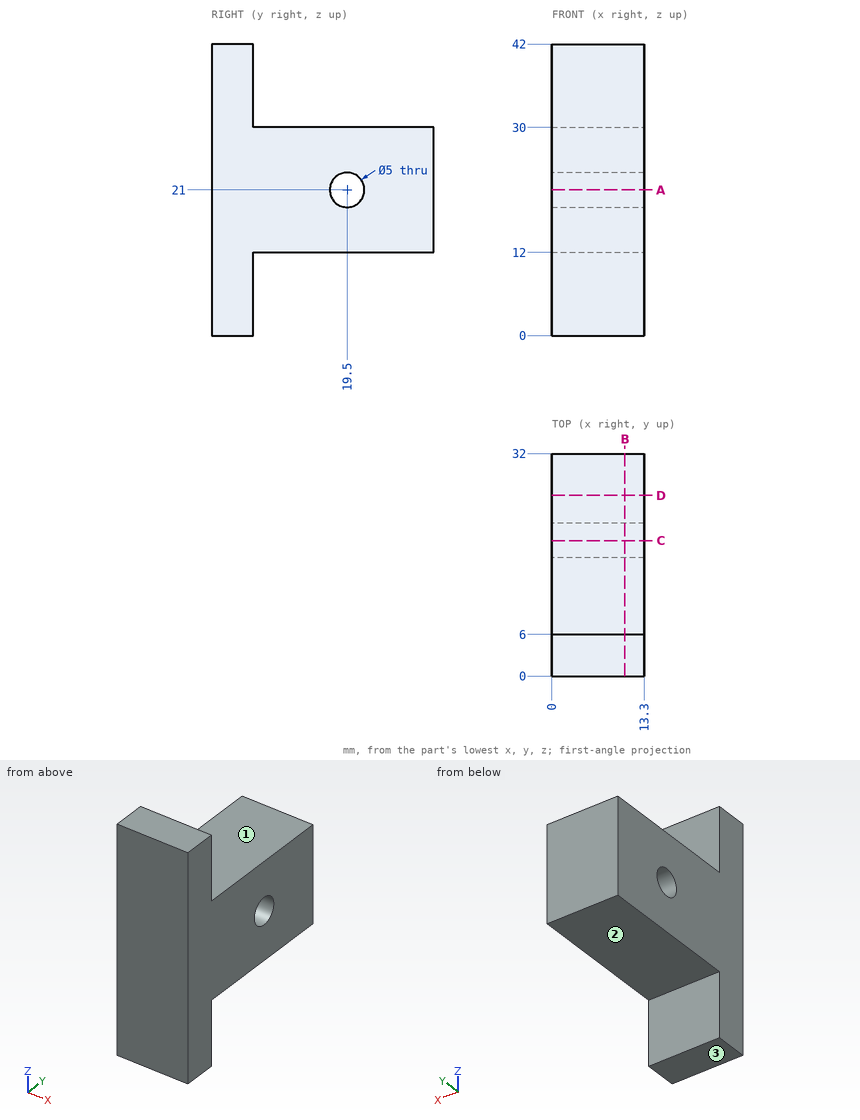
Part print with two shaded views. Sizes in mm from the minimum x, y, z corner. A direction names the side the tool comes from. Coordinates: 2 decimals unless noted, no trailing zeros. Write each loop counter-clockwise with the first axis right and the second up, starting at its lowest first coordinate (ties: lowest second). Pieces come first, ordered by that corner, then holes.
1. Band-saw the part on B-B, the plane x = 10.5. Give the cut face in (y, z).
Answer block:
outline: (0, 0) - (6, 0) - (6, 12) - (32, 12) - (32, 30) - (6, 30) - (6, 42) - (0, 42) - close; hole circle Ø5 at (19.5, 21)
2. Band-saw the part on A-A, the plane z = 21. Give the cut face in (x, y).
Answer block:
outline: (0, 0) - (13.3, 0) - (13.3, 17) - (0, 17) - close; (0, 22) - (13.3, 22) - (13.3, 32) - (0, 32) - close
3. Drop flat-ended pins along their axis: pin 1 (4 mm diameter, centred on y = 24.5, z = 33, fed in from -X); pin 2 (6 mm diameter, centred on x = 11.5, y = 10.5, fed in from +Z); pin 3 (1 mm diameter, centred on x = 2, y = 10, fed in from -Z); pin 4 (3.5 mm diameter, centred on x = 9.5, z = 4, fed in from +Y). Give the stop position or say it passes through.
Answer block:
pin 1: passes through
pin 2: stops at z = 30
pin 3: stops at z = 12
pin 4: stops at y = 6
4. 3-axis set-ups, long thin cutter, end or side, ignore diameter. For the marked faces 1, 2 and 3: which of +Z, -Z, +X, -X, +Y, -Y reach the whole face in a straight line?
Answer block:
face 1: +Z, +X, -X, +Y
face 2: -Z, +X, -X, +Y
face 3: -Z, +X, -X, +Y, -Y
5. Band-saw the part on C-C, the plane y = 19.5. Give the cut face in (x, z), and give its area (3 significant figures).
Answer block:
outline: (0, 12) - (13.3, 12) - (13.3, 18.5) - (0, 18.5) - close; (0, 23.5) - (13.3, 23.5) - (13.3, 30) - (0, 30) - close
area: 173 mm2
6. Drill centre lines: probe 1 along Y at (x, z) = (6.75, 21); probe 2 along Y at (x, z) = (5.5, 2); probe 3 along Z at (x, y) = (1, 25). Where is each one in solid material? Low to high.
Answer block:
probe 1: y = 0 to 17, 22 to 32
probe 2: y = 0 to 6
probe 3: z = 12 to 30
7. Band-saw the part on D-D, the plane y = 26. Give the cut face in (x, z).
Answer block:
outline: (0, 12) - (13.3, 12) - (13.3, 30) - (0, 30) - close
